from build123d import *

# Parameters (mm, degrees)
SKETCH_1_W          = 12
SKETCH_1_H          = 10
EXTRUDE_1_DEPTH     = 1
SKETCH_2_R          = 1
EXTRUDE_2_DEPTH     = 8
SKETCH_3_R          = 2
EXTRUDE_3_DEPTH     = 1
EXTRUDE_4_DEPTH     = 10
SKETCH_5_W          = 12
SKETCH_5_H          = 10
EXTRUDE_5_DEPTH     = 15
CUT_EXTRUDE_1_REACH = 14
SKETCH_6_R          = 0.5


with BuildPart() as part:
    # 草图1 → 凸台-拉伸1 (new body)
    with BuildSketch(Plane.XY):
        Rectangle(SKETCH_1_W, SKETCH_1_H)
    extrude(amount=EXTRUDE_1_DEPTH)

    # 草图2 → 凸台-拉伸2 (add)
    with BuildSketch(Plane(origin=(0, 0, 0), x_dir=(-1, 0, 0), z_dir=(0, 0, -1))):
        with Locations((-4.5, 3.5)):
            Circle(SKETCH_2_R)
        with Locations((4.5, 3.5)):
            Circle(SKETCH_2_R)
        with Locations((4.5, -3.5)):
            Circle(SKETCH_2_R)
        with Locations((-4.5, -3.5)):
            Circle(SKETCH_2_R)
    extrude(amount=EXTRUDE_2_DEPTH)

    # 草图3 → 凸台-拉伸3 (add)
    with BuildSketch(Plane.XY.offset(1)):
        Circle(SKETCH_3_R)
    extrude(amount=EXTRUDE_3_DEPTH)

    # 草图4 → 凸台-拉伸4 (add)
    with BuildSketch(Plane.XY.offset(2)):
        with BuildLine():
            Line((-1.118033989, 1), (1.118033989, 1))
            ThreePointArc((1.118033989, 1), (0, -1.5), (-1.118033989, 1))
        make_face()
    extrude(amount=EXTRUDE_4_DEPTH)

    # 草图5 → 凸台-拉伸5 (add)
    with BuildSketch(Plane(origin=(0, 0, -8), x_dir=(-1, 0, 0), z_dir=(0, 0, -1))):
        Rectangle(SKETCH_5_W, SKETCH_5_H)
    extrude(amount=EXTRUDE_5_DEPTH)

    # 草图6 → 切除-拉伸1 (cut, up to next)
    with BuildSketch(Plane(origin=(0, 0, 0), x_dir=(-1, 0, 0), z_dir=(0, 0, -1)), mode=Mode.PRIVATE) as cut_extrude_1_sk1:
        with Locations((-4.5, 0)):
            Circle(SKETCH_6_R)
    cut_extrude_1_tool1 = extrude(cut_extrude_1_sk1.sketch, amount=-CUT_EXTRUDE_1_REACH, mode=Mode.PRIVATE) & part.part
    add(cut_extrude_1_tool1.solids().sort_by_distance((4.5, 0, 0))[0], mode=Mode.SUBTRACT)
    # 草图6 → 切除-拉伸1 (cut, up to next)
    with BuildSketch(Plane(origin=(0, 0, 0), x_dir=(-1, 0, 0), z_dir=(0, 0, -1)), mode=Mode.PRIVATE) as cut_extrude_1_sk2:
        with Locations((4.5, 0)):
            Circle(SKETCH_6_R)
    cut_extrude_1_tool2 = extrude(cut_extrude_1_sk2.sketch, amount=-CUT_EXTRUDE_1_REACH, mode=Mode.PRIVATE) & part.part
    add(cut_extrude_1_tool2.solids().sort_by_distance((-4.5, 0, 0))[0], mode=Mode.SUBTRACT)


solid = part.part
Here's how the part is built. I have some questions about the finished solid (model axes, mm). A direction names the side the tool comes from. Round coordinates to 2 decimals unless told otherwise and drop trailing zeros. Write each loop counter-clockwise with the first axis right and the second up, starting at its lowest first coordinate (ties: lowest second). Pieces come first, ordered by that corner, then holes.
1. Will these pins go through, and if not, where does the flat tip stop? pin 1 Ø1.5 at (y, z) = (3, -2.5) entering from +X; pin 2 Ø1.1 at (x, z) = (0, 5) entering from +Y.
2. For faces 4 (the flat face through (-0.1, -5, 0.5)), 5 (the cylindrical face through (-0.434, -1.952, 1.493)), 6 (the flat face through (6, -0.1, 0.5)), 7 (the flat face through (0, 1, 7)), 8 (the flat face through (0, 0, -8)), which set-ups out of +Z, -Z, +X, -X, +Y, -Y let a thin tool reach every point of the face, with its end or its side?
3. I need wall thicknesses on L1, parallel to Z at x = 5.25, y = 1.75; L2, parallel to Y at x = 4.5, z = 0.75; L3, parallel to Z at x = -0.25, y = -1. Which ranges of each line are inside material? Lowest first, please.
4. Suppose I cut it at B-B (x = 0). List the corners of the cut face in (y, z) for me, and give its area (3 significant figures).
5. If we mould it in two halves opening along Z, with no side actions, what happens to faces 1 (the cylindrical face through (4.63, 4.49, -3.94)), 2 (the flat face through (0, 0, 12)), 3 (the flat face through (-6, 0, -15))? For each: released by +Z, released by -Z, zero draft, split by the parting line, or undercut.
6. Suppose I cut it at A-A (y = 0). List the corners of the cut face in (x, z) for me, and give its area (3 significant figures).
7. Suppose I cut it at D-D (y = -3.5). List the corners of the cut face in (x, z) for me, and give its area (3 significant figures).
8. Suppose I cut it at C-C (z = -2.5). List the corners of the cut face in (x, y) for me, and give its area (3 significant figures).
Answer sheet:
1. pin 1: stops at x = 5.5
1. pin 2: stops at y = 1
2. face 4: +Z, -Z, +X, -X, -Y
2. face 5: +Z
2. face 6: +Z, -Z, +X, +Y, -Y
2. face 7: +Z, +X, -X, +Y
2. face 8: none
3. L1: z = -23 to -8, 0 to 1
3. L2: y = -5 to -0.5, 0.5 to 5
3. L3: z = -23 to -8, 0 to 12
4. outline: (-5, -23) - (5, -23) - (5, -8) - (-5, -8) - close; (-5, 0) - (5, 0) - (5, 1) - (2, 1) - (2, 2) - (1, 2) - (1, 12) - (-1.5, 12) - (-1.5, 2) - (-2, 2) - (-2, 1) - (-5, 1) - close
4. area: 189 mm2
5. face 1: undercut
5. face 2: released by +Z
5. face 3: zero draft
6. outline: (-6, -23) - (6, -23) - (6, -8) - (-6, -8) - close; (-6, 0) - (-5, 0) - (-5, 1) - (-6, 1) - close; (-4, 0) - (4, 0) - (4, 1) - (2, 1) - (2, 2) - (1.5, 2) - (1.5, 12) - (-1.5, 12) - (-1.5, 2) - (-2, 2) - (-2, 1) - (-4, 1) - close; (5, 0) - (6, 0) - (6, 1) - (5, 1) - close
6. area: 224 mm2
7. outline: (-6, -23) - (6, -23) - (6, -8) - (5.5, -8) - (5.5, 0) - (6, 0) - (6, 1) - (-6, 1) - (-6, 0) - (-5.5, 0) - (-5.5, -8) - (-6, -8) - close; hole (-3.5, -8) - (3.5, -8) - (3.5, 0) - (-3.5, 0) - close
7. area: 224 mm2
8. outline: circle Ø2 at (-4.5, -3.5); circle Ø2 at (-4.5, 3.5); circle Ø2 at (4.5, -3.5); circle Ø2 at (4.5, 3.5)
8. area: 12.6 mm2
